from build123d import *

# Parameters (mm, degrees)
F1_DEPTH   = 500
F2_W       = 25.3097712994
F2_H       = 27.039706707
F1_FACE1_W = 54.7773372423
F1_FACE1_H = 500
F3_DEPTH   = 189.0395001898
F4_W       = 25.3097712994
F4_H       = 27.051
F5_DEPTH   = 189.0395001898


with BuildPart() as f1:
    # F0 (on Front) → F1 (new body)
    with BuildSketch(Plane.XZ):
        Polygon((29.4588804245, 0), (0, 0), (0, -211.5057110786), (54.7686517239, -212.4811410904), (54.7686517239, -64.9340748787), (54.7686517239, -23.4426409006), (29.4588804245, -23.4426409006), align=None)
    extrude(amount=F1_DEPTH)

    # F2 (on face) + F1_face1 (on face) → F3 (cut, through all)
    with BuildSketch(Plane.XY.offset(-23.4426409006)):
        with Locations((42.1137660742, -13.5198533535)):
            Rectangle(F2_W, F2_H)
    with BuildSketch(Plane(origin=(27.3843258619, -250, -211.9934260845), x_dir=(1, 0, 0), z_dir=(-0.017807182, 0, -0.9998414396))):
        Rectangle(F1_FACE1_W, F1_FACE1_H)
    extrude(amount=-F3_DEPTH, dir=(0, 0, 1), mode=Mode.SUBTRACT)

    # F4 (on face) → F5 (cut, through all)
    with BuildSketch(Plane.XY.offset(-23.4426409006)):
        with Locations((42.1137660742, -486.4745)):
            Rectangle(F4_W, F4_H)
    extrude(amount=-F5_DEPTH, mode=Mode.SUBTRACT)


solid = f1.part
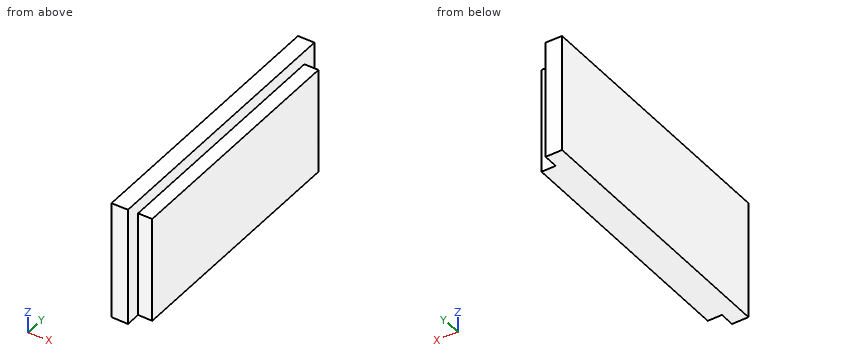
Read the model definition and answer for the solid it produces. Units are mm, in the model's axes. Coordinates: 2 decimals unless noted, no trailing zeros. Loops run counter-clockwise (first coordinate to the right, second up) from the corner with the lowest first, then second, coordinate; pieces in that order, holes last. Notation, with made-up numbers: (66, -2) -> (117, -2) arc R18 cw to (117, 3) -> close; hole circle Ø5 at (50, 38.25). An arc over 180 degrees is marked (long way). Answer in a Markdown table with one row per item.
Item 1: Straight lines are drawn through the part: line 1 along Z through (x, y) = (33.5, -350); line 2 along Z through (x, y) = (30, -426.5); line 3 along Y through (x, z) = (32, -188). For each, find the intervals that lie inside material, in ascending order. Write a range as [from, to].
Returned:
| item | result |
|---|---|
| line 1 | z = [-212.1, -23.44] |
| line 2 | z = [-212.04, -23.44] |
| line 3 | y = [-472.95, -27.04] |
Item 2: Each of these flat-tipped pins is pushed along its axis until it touches: P1, Ø7.5, axis at x = 42.5, y = -162.5, coming from the +Z side; P2, Ø20, axis at x = 48, z = -98.5, coming from the +Y side; P3, Ø10, axis at x = 10, y = -66.5, coming from the -Z side. Where does it stop, or does it pass through?
Returned:
| item | result |
|---|---|
| P1 | stops at z = -23.44 |
| P2 | stops at y = -27.04 |
| P3 | stops at z = -211.77 |
Item 3: A cutting plane is placed at C-C on x = 36. Determine the outline of the cut face in (y, z), plus the area to 3 significant figures.
Returned:
| item | result |
|---|---|
| outline | (-472.95, -212.15) -> (-27.04, -212.15) -> (-27.04, -23.44) -> (-472.95, -23.44) -> close |
| area | 84,100 mm^2 |
Item 4: A cutting plane is placed at B-B on y = -359.5. Determine the outline of the cut face in (x, z), plus the area to 3 significant figures.
Returned:
| item | result |
|---|---|
| outline | (0, -211.51) -> (54.77, -212.48) -> (54.77, -23.44) -> (29.46, -23.44) -> (29.46, 0) -> (0, 0) -> close |
| area | 11,000 mm^2 |
Item 5: A cutting plane is placed at A-A on z = -81.5. Determine the outline of the cut face in (x, y), plus the area to 3 significant figures.
Returned:
| item | result |
|---|---|
| outline | (0, -500) -> (29.46, -500) -> (29.46, -472.95) -> (54.77, -472.95) -> (54.77, -27.04) -> (29.46, -27.04) -> (29.46, 0) -> (0, 0) -> close |
| area | 26,000 mm^2 |
